Geometry check sheet. Reference: the model listing, model coordinates, mm. Coordinates: 2 decimals unless noted, no trailing zeros. Write each loop counter-clockwise with the first axis right and the second up, starting at its lowest first coordinate (ties: lowest second). Pieces come first, ordered by that corner, then holes. Notation, with made-up numbers: (22, 61) -> (62, 61) arc R25 cw to (62, 88) -> close; hole circle Ø11 at (88.25, 14.5). An arc over 180 degrees is marked (long way). Answer in a Markdown table with one row per item. Add a question column.
Q1. Section check B-B, the plane y = 12.5. Record the boundary of the cut face in (x, z), and give its area (3 significant figures).
Q2. Section check D-D, the plane z = 2.2. Count the separate pieces of the cut face and the enclosed holes in it, and give its area (3 significant figures).
Q3. Thickness scan on line 1 (Y direction, x = 27.5, z = 0.7); line 2 (X direction, y = 9, z = 0.3); line 3 (Y direction, x = -27.5, z = 1.4). Record the ranges inside material, lowest first.
Q4. Section check A-A, the plane x = 27.5. Record the boundary of the cut face in (y, z), and give its area (3 significant figures).
Q5. Section check C-C, the plane x = 11. Record the boundary of the cut face in (y, z), and give its area (3 significant figures).
Q6. Gauge pin test, flat end, axial feed: P1, Ø0.8, axis at x = -37.5, z = 1.5, coming from the -Y side. Record the tip position at first contact, or that the pin passes through.
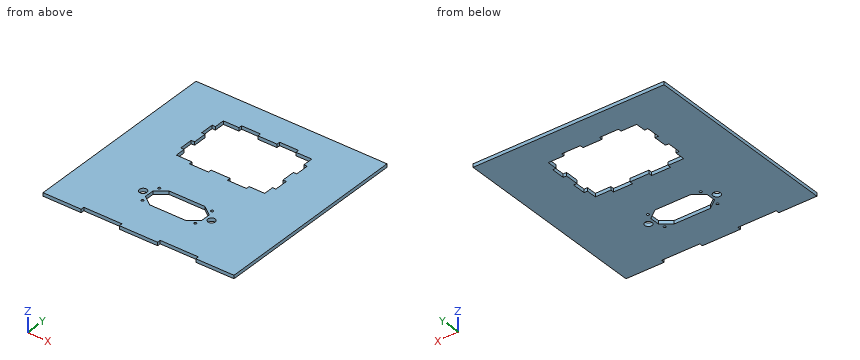
```python
from build123d import *

# Parameters (mm, degrees)
SKETCH1_R           = 1
SKETCH1_R_2         = 3
SKETCH1_R_3         = 2.9
BOSS_EXTRUDE3_DEPTH = 2.7


with BuildPart() as part:
    # Sketch1 → Boss-Extrude3 (new body)
    with BuildSketch(Plane.XY):
        Polygon((-46.02, -28), (-46.02, -25.3), (-15.34, -25.3), (-15.34, -28), (15.34, -28), (15.34, -25.3), (46.02, -25.3), (46.02, -28), (76.7, -28), (76.7, -25.3), (76.7, -23), (76.7, 13), (76.7, 131.5), (-76.7, 131.5), (-76.7, 13), (-76.7, -23), (-76.7, -25.3), (-76.7, -28), align=None)
        with Locations((-21.25, 3.75)):
            Circle(SKETCH1_R, mode=Mode.SUBTRACT)
        with Locations((-27.5, 12.5)):
            Circle(SKETCH1_R_2, mode=Mode.SUBTRACT)
        with Locations((-21.25, 21.25)):
            Circle(SKETCH1_R, mode=Mode.SUBTRACT)
        with Locations((21.25, 3.75)):
            Circle(SKETCH1_R, mode=Mode.SUBTRACT)
        with Locations((27.5, 12.5)):
            Circle(SKETCH1_R_3, mode=Mode.SUBTRACT)
        with Locations((21.25, 21.25)):
            Circle(SKETCH1_R, mode=Mode.SUBTRACT)
        Polygon((-22.5, 16.5), (-14.5, 22.5), (14.5, 22.5), (22.5, 16.5), (22.5, 8.5), (14.5, 2.5), (0, 2.5), (-14.5, 2.5), (-22.5, 8.5), align=None, mode=Mode.SUBTRACT)
        Polygon((35.5, 57.5), (22.92, 57.5), (22.92, 54.8), (7.64, 54.8), (7.64, 57.5), (-7.64, 57.5), (-7.64, 54.8), (-22.92, 54.8), (-22.92, 57.5), (-35.5, 57.5), (-35.5, 65.68), (-38.2, 65.68), (-38.2, 76.56), (-35.5, 76.56), (-35.5, 87.44), (-38.2, 87.44), (-38.2, 98.32), (-35.5, 98.32), (-35.5, 106.5), (-22.92, 106.5), (-22.92, 109.2), (-7.64, 109.2), (-7.64, 106.5), (7.64, 106.5), (7.64, 109.2), (22.92, 109.2), (22.92, 106.5), (35.5, 106.5), (35.5, 98.32), (38.2, 98.32), (38.2, 87.44), (35.5, 87.44), (35.5, 76.56), (38.2, 76.56), (38.2, 65.68), (35.5, 65.68), align=None, mode=Mode.SUBTRACT)
    extrude(amount=BOSS_EXTRUDE3_DEPTH)


solid = part.part
```
Calculated:
| question | item | result |
|---|---|---|
| 1 | outline | (-76.7, 0) -> (-30.5, 0) -> (-30.5, 2.7) -> (-76.7, 2.7) -> close; (-24.5, 0) -> (-22.5, 0) -> (-22.5, 2.7) -> (-24.5, 2.7) -> close; (22.5, 0) -> (24.6, 0) -> (24.6, 2.7) -> (22.5, 2.7) -> close; (30.4, 0) -> (76.7, 0) -> (76.7, 2.7) -> (30.4, 2.7) -> close |
| 1 | area | 261 mm² |
| 2 | separate pieces | 1 |
| 2 | enclosed holes | 8 |
| 2 | area | 19,700 mm² |
| 3 | line 1 | y = -25.3 to 9.6, 15.4 to 57.5, 106.5 to 131.5 |
| 3 | line 2 | x = -76.7 to -22.5, 22.5 to 76.7 |
| 3 | line 3 | y = -25.3 to 9.5, 15.5 to 57.5, 106.5 to 131.5 |
| 4 | outline | (-25.3, 0) -> (9.6, 0) -> (9.6, 2.7) -> (-25.3, 2.7) -> close; (15.4, 0) -> (57.5, 0) -> (57.5, 2.7) -> (15.4, 2.7) -> close; (106.5, 0) -> (131.5, 0) -> (131.5, 2.7) -> (106.5, 2.7) -> close |
| 4 | area | 275 mm² |
| 5 | outline | (-28, 0) -> (2.5, 0) -> (2.5, 2.7) -> (-28, 2.7) -> close; (22.5, 0) -> (54.8, 0) -> (54.8, 2.7) -> (22.5, 2.7) -> close; (109.2, 0) -> (131.5, 0) -> (131.5, 2.7) -> (109.2, 2.7) -> close |
| 5 | area | 230 mm² |
| 6 | P1 | stops at y = -25.3 |
